Autodesk Inventor part; units mm, degrees
ref_plane "YZ Plane" through (0, 0, 0) normal (1, 0, 0) x (0, 1, 0)
ref_plane "XZ Plane" through (0, 0, 0) normal (0, 1, 0) x (-1, 0, 0)
ref_plane "XY Plane" through (0, 0, 0) normal (0, 0, 1) x (1, 0, 0)
sketch "Sketch1" plane through (0, 0, 0) normal (0, 1, 0) x (-1, 0, 0)
  circle A0 centre (0, 0) radius 26.543
  dimension "d0" = 53.086
extrude "Extrusion1" add sketch "Sketch1" along normal blind 16.3068
sketch "Sketch2" plane through (0, 16.3068, 0) normal (0, 1, 0) x (1, 0, 0)
  circle A0 centre (0, 0) radius 23.495
  dimension "d3" = 46.99
extrude "Extrusion2" cut sketch "Sketch2" against normal blind 12.7
sketch "Sketch3" plane through (0, 16.3068, 0) normal (0, 1, 0) x (1, 0, 0)
  circle A0 centre (0, 0) radius 31.623
  circle A1 centre (0, 0) radius 23.401
  dimension "d6" = 63.246
extrude "Extrusion4" add sketch "Sketch3" along normal blind 2.1082
fillet "Fillet2" radius 1.524 1 edges at (-23.495, 3.6068, 0)
fillet "Fillet3" radius 2 1 edges at (26.543, 0, 0)
properties part number "_3DPrint"
CAD build for the part. Positions are in the model's coordinates, mm. A direction names the side the tool comes from. Coordinates: 2 decimals unless noted, no trailing zeros. Write each loop counter-clockwise with the first axis right and the second up, starting at its lowest first coordinate (ties: lowest second). Pieces come first, ordered by that corner, then holes. Notation, with made-up numbers: M -1.75,16.25 L 30.25,16.25 A22 cw 30.25,35.25 Z; hole C -11.75,7 d7. An arc over 180 degrees is marked long. Return JSON: item names as keys, results as strings.
Item 1: Probe line 1 (Z direction, x = 0, y = 8) (3 decimals); line 2 (X direction, y = 17.8, z = 0). List the from-to ranges inside material, lowest first. Write a range as from..to.
Findings below:
{"line 1": "z = -26.543..-23.495, 23.495..26.543", "line 2": "x = -31.62..-23.4, 23.4..31.62"}
Item 2: Slice it at C-C, the plane z = 0. Write the cut outline in (x, y) (3 decimals), and give its area (3 significant figures).
Findings below:
{"outline": "M -31.623,16.307 L -26.543,16.307 L -26.543,2 A2 ccw -24.543,0 L 24.543,0 A2 ccw 26.543,2 L 26.543,16.307 L 31.623,16.307 L 31.623,18.415 L 23.401,18.415 L 23.401,16.307 L 23.495,16.307 L 23.495,5.131 A1.524 cw 21.971,3.607 L -21.971,3.607 A1.524 cw -23.495,5.131 L -23.495,16.307 L -23.401,16.307 L -23.401,18.415 L -31.623,18.415 Z", "area": "303 mm2"}
Item 3: Slice it at B-B, the plane y = 12. Write the cut outline in (x, z) (3 decimals), and give its area (3 significant figures).
Findings below:
{"outline": "C 0,0 d53.086; hole C 0,0 d46.99", "area": "479 mm2"}
Item 4: Two-plate mould, pull along Z, no slides. Class faces 1 (the flat face through (0, 3.607, 0)), 2 (the flat face through (-7, 16.307, -26)), 3 (the cylindrical face through (-25.095, 17.346, -19.242)): +Z half, -Z half, draft (parallel to the pull), parting line (faces both ways), or undercut.
Findings below:
{"face 1": "undercut", "face 2": "draft", "face 3": "parting line"}
Item 5: Drop flat-ended pins along their axis: pin 1 Ø3 at (y, z) = (10, -13) entering from -X; pin 2 Ø1 at (x, y) = (-11.5, 2.5) entering from +Z; pin 3 Ø2 at (x, y) = (11, 12) entering from -Z. Give the stop position or say it passes through.
Findings below:
{"pin 1": "stops at x = -23.92", "pin 2": "stops at z = 24.16", "pin 3": "stops at z = -24.59"}
Item 6: Which spindle directions (+Z, -Z, +X, -X, +Y, -Y) get a long thin tool onto all of the face, cutting with end or side? Do faces 4 (the cylindrical face through (21.6, 17.3, -9)), 5 (the cylindrical face through (-5.093, 10.797, 22.936)), 6 (the cylindrical face through (-12.248, 9.053, 23.548)), 7 (the flat face through (0, 0, 0)). Say none if no direction does.
Findings below:
{"face 4": "+Y", "face 5": "none", "face 6": "-Y", "face 7": "+Z, -Z, +X, -X, -Y"}
Item 7: Slice it at A-A, the plane x = 0. Write the cut outline in (y, z) (3 decimals).
Findings below:
{"outline": "M 0,-24.543 A2 ccw 2,-26.543 L 16.307,-26.543 L 16.307,-31.623 L 18.415,-31.623 L 18.415,-23.401 L 16.307,-23.401 L 16.307,-23.495 L 5.131,-23.495 A1.524 cw 3.607,-21.971 L 3.607,21.971 A1.524 cw 5.131,23.495 L 16.307,23.495 L 16.307,23.401 L 18.415,23.401 L 18.415,31.623 L 16.307,31.623 L 16.307,26.543 L 2,26.543 A2 ccw 0,24.543 Z"}
